Part model, mm, in its own coordinate system. A direction names the side the tool comes from. Round coordinates to 2 decimals unless told otherwise and drop trailing zeros. Write each loop counter-clockwise with the first axis right and the second up, starting at its lowest first coordinate (ties: lowest second). Pieces come first, ordered by that corner, then holes. Notation, with made-up numbers: (67.5, 13) -> (110.5, 13) arc R33 cw to (110.5, 51) -> close; hole circle Ø9 at (36, 58.5). An arc over 180 degrees is marked (long way). Return JSON: item names as keys, results as strings. Group by question number.
(1) Mould opens along Z. For faces 1 (the flat face through (48, -12, 13)), 2 (the cylindrical face through (-22.21, -5.92, -53.58)), 3 (the cylindrical face through (52.29, -6.08, 0.38)) say: +Z half, -Z half, draft (parallel to the pull), parting line (faces both ways), or undercut.
(2) Saw through at C-C (z = 54). List the corners of the cut face in (x, y).
(3) Saw through at D-D (x = -54). List the corners of the cut face in (y, z), plus the area to 3 significant figures.
(4) Tool access for faces 4 (the flat face through (43, 0, -26)), 5 (the cylindrical face through (-43.028, -5.916, -22.38)), 6 (the cylindrical face through (-0.67, -6.084, -55.617)): list every direction of +Z, -Z, +X, -X, +Y, -Y with a clear straight run to the whole face (end or side of a thin tool).
(5) Saw through at A-A (z = 0). List the corners of the cut face in (x, y), plus the area to 3 significant figures.
(6) Drop flat-ended pins along their axis: pin 1 Ø3 at (y, z) = (29.5, -20.5) entering from -X; pin 2 Ø12 at (x, y) = (-43, 6.5) entering from +Z; pin 3 Ø10 at (y, z) = (15.5, -10) entering from +X; pin 4 Ø3 at (x, z) = (0, 54) entering from +Y. Give the stop position or say it passes through.
(7) Drill centre lines: L1, parallel to X at y = -8, z = 0; L2, parallel to Y at x = 35, z = -42; L3, parallel to X at y = 26, z = 19. Where is each one in solid material? Low to high. Write a range as from..to.
(8) Saw through at B-B (x = 0). List the corners of the cut face in (y, z).
from build123d import *

# Parameters (mm, degrees)
CUT_EXTRUDE1_REACH  = 86.879
SKETCH2_R           = 12
SKETCH3_R           = 58
SKETCH3_R_2         = 48.5
BOSS_EXTRUDE1_DEPTH = 12
CUT_EXTRUDE2_REACH  = 103.627
SKETCH4_R           = 1.75


with BuildPart() as part:
    # Sketch1 → Revolve-Thin1 (revolve)
    with BuildSketch(Plane.XY, mode=Mode.PRIVATE) as revolve_thin1_sk:
        with BuildLine():
            Line((0, 47), (11.968709204, 47))
            ThreePointArc((11.968709204, 47), (38.293161246, 29.763800191), (48.5, 0))
            Line((48.5, 0), (49.5, 0))
            ThreePointArc((49.5, 0), (39.044030516, 30.427186546), (12.093386622, 48))
            Line((12.093386622, 48), (0, 48))
            Line((0, 48), (0, 47))
        make_face()
    revolve(revolve_thin1_sk.sketch.rotate(Axis((0, -100.538171033, 0), (0, 1, 0)), 90), axis=Axis((0, -100.538171033, 0), (0, 1, 0)))

    # Sketch2 → Cut-Extrude1 (cut, up to next)
    with BuildSketch(Plane(origin=(0, 48, 0), x_dir=(1, 0, 0), z_dir=(0, 1, 0)), mode=Mode.PRIVATE) as cut_extrude1_sk1:
        with Locations(Location((0, 0, 0), (0, 0, 270))):
            Circle(SKETCH2_R)
    cut_extrude1_tool1 = extrude(cut_extrude1_sk1.sketch, amount=-CUT_EXTRUDE1_REACH, mode=Mode.PRIVATE) & part.part
    add(cut_extrude1_tool1.solids().sort_by_distance((0, 48, 0))[0], mode=Mode.SUBTRACT)

    # Sketch3 → Boss-Extrude1 (add)
    with BuildSketch(Plane.XZ):
        with Locations(Location((0, 0, 0), (0, 0, 270))):
            Circle(SKETCH3_R)
        with Locations(Location((0, 0, 0), (0, 0, 270))):
            Circle(SKETCH3_R_2, mode=Mode.SUBTRACT)
    extrude(amount=BOSS_EXTRUDE1_DEPTH)

    # Sketch4 → Cut-Extrude2 (cut, up to next)
    with BuildSketch(Plane.XZ.offset(12), mode=Mode.PRIVATE) as cut_extrude2_sk1:
        with Locations(Location((0, 54, 0), (0, 0, 270))):
            Circle(SKETCH4_R)
    cut_extrude2_tool1 = extrude(cut_extrude2_sk1.sketch, amount=-CUT_EXTRUDE2_REACH, mode=Mode.PRIVATE) & part.part
    # Sketch4 → Cut-Extrude2 (cut, up to next)
    with BuildSketch(Plane.XZ.offset(12), mode=Mode.PRIVATE) as cut_extrude2_sk2:
        with Locations(Location((54, 0, 0), (0, 0, 270))):
            Circle(SKETCH4_R)
    cut_extrude2_tool2 = extrude(cut_extrude2_sk2.sketch, amount=-CUT_EXTRUDE2_REACH, mode=Mode.PRIVATE) & part.part
    # Sketch4 → Cut-Extrude2 (cut, up to next)
    with BuildSketch(Plane.XZ.offset(12), mode=Mode.PRIVATE) as cut_extrude2_sk3:
        with Locations(Location((-54, 0, 0), (0, 0, 270))):
            Circle(SKETCH4_R)
    cut_extrude2_tool3 = extrude(cut_extrude2_sk3.sketch, amount=-CUT_EXTRUDE2_REACH, mode=Mode.PRIVATE) & part.part
    # Sketch4 → Cut-Extrude2 (cut, up to next)
    with BuildSketch(Plane.XZ.offset(12), mode=Mode.PRIVATE) as cut_extrude2_sk4:
        with Locations(Location((0, -54, 0), (0, 0, 270))):
            Circle(SKETCH4_R)
    cut_extrude2_tool4 = extrude(cut_extrude2_sk4.sketch, amount=-CUT_EXTRUDE2_REACH, mode=Mode.PRIVATE) & part.part
    add(cut_extrude2_tool1.solids().sort_by_distance((0, -12, 54))[0], mode=Mode.SUBTRACT)
    add(cut_extrude2_tool2.solids().sort_by_distance((54, -12, 0))[0], mode=Mode.SUBTRACT)
    add(cut_extrude2_tool3.solids().sort_by_distance((-54, -12, 0))[0], mode=Mode.SUBTRACT)
    add(cut_extrude2_tool4.solids().sort_by_distance((0, -12, -54))[0], mode=Mode.SUBTRACT)


solid = part.part
Computed values:
{
 "1": {"face 1": "draft", "face 2": "parting line", "face 3": "undercut"},
 "2": {"outline": "(-21.17, -12) -> (-1.75, -12) -> (-1.75, 0) -> (-21.17, 0) -> close; (1.75, -12) -> (21.17, -12) -> (21.17, 0) -> (1.75, 0) -> close"},
 "3": {"outline": "(-12, -21.17) -> (0, -21.17) -> (0, -1.75) -> (-12, -1.75) -> close; (-12, 1.75) -> (0, 1.75) -> (0, 21.17) -> (-12, 21.17) -> close", "area": "466 mm2"},
 "4": {"face 4": "+Y", "face 5": "-Y", "face 6": "+Y, -Y"},
 "5": {"outline": "(-58, -12) -> (-55.75, -12) -> (-55.75, 0) -> (-58, 0) -> close; (-52.25, -12) -> (-48.5, -12) -> (-48.5, 0) arc R48.5 cw to (-12, 46.99) -> (-12, 48) -> (-12.09, 48) arc R49.5 ccw to (-49.5, 0) -> (-52.25, 0) -> close; (12, 46.99) arc R48.5 cw to (48.5, 0) -> (48.5, -12) -> (52.25, -12) -> (52.25, 0) -> (49.5, 0) arc R49.5 ccw to (12.09, 48) -> (12, 48) -> close; (55.75, -12) -> (58, -12) -> (58, 0) -> (55.75, 0) -> close", "area": "274 mm2"},
 "6": {"pin 1": "x = -35.57", "pin 2": "z = 32.32", "pin 3": "x = 47.64", "pin 4": "through"},
 "7": {"L1": "-58..-55.75, -52.25..-48.5, 48.5..52.25, 55.75..58", "L2": "-12..0", "L3": "-37.59..-36.27, 36.27..37.59"},
 "8": {"outline": "(-12, -58) -> (0, -58) -> (0, -55.75) -> (-12, -55.75) -> close; (-12, -52.25) -> (0, -52.25) -> (0, -49.5) arc R49.5 ccw to (48, -12.09) -> (48, -12) -> (46.99, -12) arc R48.5 cw to (0, -48.5) -> (-12, -48.5) -> close; (-12, 48.5) -> (0, 48.5) arc R48.5 cw to (46.99, 12) -> (48, 12) -> (48, 12.09) arc R49.5 ccw to (0, 49.5) -> (0, 52.25) -> (-12, 52.25) -> close; (-12, 55.75) -> (0, 55.75) -> (0, 58) -> (-12, 58) -> close"}
}
